Check sheet for the modelled part. Datum: model origin and axes. Units: mm. Face numbers are marked on the shaded views. A direction names the side the tool comes from. Round coordinates to 2 decimals unless told otherwise and drop trailing zeros. Order: outer loops, then holes, each group sorted by start corner. A loop starts at its lowest first (then second) coordinate and runs counter-clockwise, first axis right, second up. Notation, with made-up numbers: (29.25, 73.25) -> (85.25, 73.25) arc R20 cw to (85.25, 88.25) -> close; hole circle Ø6 at (-17, 56.5). An arc over 180 degrees is marked (long way). Use CSV: the item, a comma, the result in double quotes.
```python
from build123d import *

# Parameters (mm, degrees)
F0_W     = 81
F0_H     = 53
F1_DEPTH = 35
F3_DEPTH = 81
F4_DEPTH = 81.001
F5_T     = -2
F6_DEPTH = 25


with BuildPart() as f1:
    # F0 (on Top) → F1 (new body)
    with BuildSketch(Plane.XY):
        with Locations((6.5364544774, 0)):
            Rectangle(F0_W, F0_H)
    extrude(amount=F1_DEPTH)

    # F2 (on face) → F3 (join, through all)
    with BuildSketch(Plane.YZ.offset(47.0364544774)):
        Polygon((26.5, 35), (26.5, 0), (34.5, 35), align=None)
    extrude(amount=-F3_DEPTH)

    # F2 (on face) → F4 (cut, through all)
    with BuildSketch(Plane.YZ.offset(47.0364544774)):
        Polygon((-26.5, 35), (-26.5, 0), (-18.5, 35), align=None)
    extrude(amount=-F4_DEPTH, mode=Mode.SUBTRACT)

    # F5
    f5_openings = [f1.faces().sort_by_distance(p)[0] for p in [
        (6.536454, 8, 35),
    ]]
    offset(amount=F5_T, openings=f5_openings)

    # F6 (cut): a face of the model
    f6_faces = [f1.faces().sort_by_distance(p)[0] for p in [
        (6.5364544774, 0.4571428571, 2),
    ]]
    extrude(f6_faces, amount=-F6_DEPTH, mode=Mode.SUBTRACT)


solid = f1.part
```
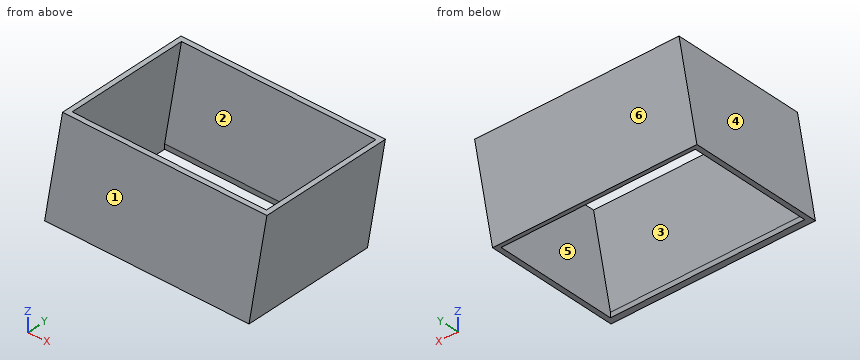
Q1. Access from +Z, -Z, +X, -X, +Y, -Y to the whole of each face (thin tool, end or side, straight path). Record for the marked faces 1, 2 and 3.
Result sheet:
face 1,"+Z, +X, -X, -Y"
face 2,"+Z"
face 3,"-Z"
Q2. Go/stop test with flat-tipped pins: pin 1 (5 mm diameter, centred on x = -19, z = 8, fed in from -Y); pin 2 (0.6 mm diameter, centred on x = -5, z = 1, fed in from -Y); pin 3 (6 mm diameter, centred on x = 31, z = 27, fed in from -Y). Record where each tip stops, or that it passes through.
Result sheet:
pin 1,"stops at y = -25.24"
pin 2,"stops at y = -26.34"
pin 3,"stops at y = -21.01"
Q3. Sectioned sample at D-D, the plane y = 30. Enter the section's corners in (x, z), then the cut area to 3 significant figures.
Result sheet:
outline,"(-33.96, 15.31) -> (47.04, 15.31) -> (47.04, 35) -> (45.04, 35) -> (45.04, 24.29) -> (-31.96, 24.29) -> (-31.96, 35) -> (-33.96, 35) -> close"
area,"770 mm^2"
Q4. Mould release check, pull along Y, two halves, no side actions. Record for the marked faces 4, 5 and 6: pulls with the +Y half, pulls with the -Y half, needs draft (parallel to the pull), parting line crosses it, or undercut.
Result sheet:
face 4,"needs draft"
face 5,"undercut"
face 6,"pulls with the +Y half"
Q5. Sectioned sample at C-C, the plane z = 27.5. Enter the section's corners in (x, y), then the cut area to 3 significant figures.
Result sheet:
outline,"(-33.96, -20.21) -> (47.04, -20.21) -> (47.04, 32.79) -> (-33.96, 32.79) -> close; hole (-31.96, -18.16) -> (45.04, -18.16) -> (45.04, 30.73) -> (-31.96, 30.73) -> close"
area,"528 mm^2"
Q6. Scan lines: L1, parallel to X at y = 13, z = 7; L2, parallel to Y at x = 1, z = 20; L3, parallel to Y at x = 3.5, z = 7. Record each from-to range of solid material in increasing order.
Result sheet:
L1,"x = -33.96 to -31.96, 45.04 to 47.04"
L2,"y = -21.93 to -19.88, 29.02 to 31.07"
L3,"y = -24.9 to -22.85, 26.05 to 28.1"
Q7. Sectioned sample at B-B, the plane x = 30.5. Enter the section's corners in (y, z), then the cut area to 3 significant figures.
Result sheet:
outline,"(-26.5, 0) -> (-23.99, 0) -> (-23.99, 2) -> (-16.45, 35) -> (-18.5, 35) -> close; (24.91, 0) -> (26.5, 0) -> (34.5, 35) -> (32.45, 35) -> (24.91, 2) -> close"
area,"144 mm^2"
Q8. Sectioned sample at A-A, the plane y = -5. Enter the section's corners in (x, z), then the cut area to 3 significant figures.
Result sheet:
outline,"(-33.96, 0) -> (-31.96, 0) -> (-31.96, 35) -> (-33.96, 35) -> close; (45.04, 0) -> (47.04, 0) -> (47.04, 35) -> (45.04, 35) -> close"
area,"140 mm^2"
